The listing builds one solid part. Answer for the finished solid, in the listing's coordinates (mm). A direction names the side the tool comes from. Give positions to 0.01 mm unless a question says otherwise; leave off trailing zeros. Order: outer loops, then holes, each group sorted by start corner. A loop starts at its lowest first (then second) coordinate and runs counter-clockwise, first axis right, second up. Notation, with made-up numbers: (-29, -27) -> (15, -27) arc R27 ccw to (15, -4) -> close; hole circle Ø3 at (31, 7). An arc over 180 degrees is marked (long way). Write item = value, one per line. Start each with the question number.
```python
from build123d import *

# Parameters (mm, degrees)
PAD_DEPTH              = 30
SKETCH001_R            = 19
SKETCH001_R_2          = 5.5
POCKET_DEPTH           = 2
LINEARPATTERN_COUNT    = 2
LINEARPATTERN_PITCH    = 24
LINEARPATTERN001_COUNT = 2
LINEARPATTERN001_PITCH = 24
FILLET_R               = 5
CHAMFER_SIZE           = 0.5
CHAMFER001_SIZE        = 1


with BuildPart() as part:
    # Sketch → Pad (new body, symmetric)
    with BuildSketch(Plane.XZ):
        with BuildLine():
            ThreePointArc((-3.872983, 5), (0, 2), (3.872983, 5))
            Line((3.872983, 5), (7.872983, 5))
            Line((7.872983, 5), (9.994304, 2.87868))
            ThreePointArc((9.994304, 2.87868), (10.837449, 0.843146), (12.872983, 0))
            Line((30, 0), (12.872983, 0))
            Line((30, -3), (30, 0))
            Line((-30, -3), (30, -3))
            Line((-30, 0), (-30, -3))
            Line((-12.872983, 0), (-30, 0))
            ThreePointArc((-12.872983, 0), (-10.837449, 0.843146), (-9.994304, 2.87868))
            Line((-7.872983, 5), (-9.994304, 2.87868))
            Line((-3.872983, 5), (-7.872983, 5))
        make_face()
    extrude(amount=PAD_DEPTH, both=True)

    # Sketch001 → Pocket (cut, symmetric)
    with BuildSketch(Plane.XZ):
        with Locations((0, 18)):
            Circle(SKETCH001_R)
        with Locations((0, 6)):
            Circle(SKETCH001_R_2, mode=Mode.SUBTRACT)
    pocket = extrude(amount=POCKET_DEPTH, both=True, mode=Mode.SUBTRACT)

    # LinearPattern: Pocket ×2
    with Locations(*[(0, -i * LINEARPATTERN_PITCH, 0) for i in range(1, LINEARPATTERN_COUNT)]):
        add(pocket, mode=Mode.SUBTRACT)

    # LinearPattern001: Pocket ×2
    with Locations(*[(0, i * LINEARPATTERN001_PITCH, 0) for i in range(1, LINEARPATTERN001_COUNT)]):
        add(pocket, mode=Mode.SUBTRACT)

    # Fillet
    fillet_edges = [part.edges().sort_by_distance(p)[0] for p in [
        (30, -30, -1.5),
        (30, 30, -1.5),
        (-30, -30, -1.5),
        (-30, 30, -1.5),
    ]]
    fillet(fillet_edges, radius=FILLET_R)

    # Chamfer
    chamfer_edges = [part.edges().sort_by_distance(p)[0] for p in [
        (-5.872983, 30, 5),
        (-7.872983, 28, 5),
        (-6.640655, 26, 5),
        (-5.408327, 24, 5),
        (-6.640655, 22, 5),
        (-7.872983, 12, 5),
        (-6.640655, 2, 5),
        (-5.408327, 0, 5),
        (-6.640655, -2, 5),
        (-7.872983, -12, 5),
        (-6.640655, -22, 5),
        (-5.408327, -24, 5),
        (-6.640655, -26, 5),
        (-7.872983, -28, 5),
        (-5.872983, -30, 5),
        (-3.872983, 0, 5),
        (5.872983, 30, 5),
        (7.872983, 28, 5),
        (6.640655, 26, 5),
        (5.408327, 24, 5),
        (6.640655, 22, 5),
        (7.872983, 12, 5),
        (6.640655, 2, 5),
        (5.408327, 0, 5),
        (6.640655, -2, 5),
        (7.872983, -12, 5),
        (6.640655, -22, 5),
        (5.408327, -24, 5),
        (6.640655, -26, 5),
        (7.872983, -28, 5),
        (5.872983, -30, 5),
        (3.872983, 0, 5),
    ]]
    chamfer(chamfer_edges, length=CHAMFER_SIZE)

    # Chamfer001
    chamfer001_edges = [part.edges().sort_by_distance(p)[0] for p in [
        (18.936492, -30, 0),
        (-18.936492, -30, 0),
    ]]
    chamfer(chamfer001_edges, length=CHAMFER001_SIZE)


solid = part.part
```
Item 1: Consider L1, parallel to Y at x = -1, z = -0.75; L2, parallel to X at y = 23, z = 1.5; L3, parallel to Z at x = 22, y = -2. Determine where each line is inside the solid, lowest interval first. Write a range as from..to.
Item 2: A cutting plane is placed at B-B, the plane y = -15.5. Write down the section's boundary in (x, z), plus the area to 3 significant figures.
Item 3: Which of the six approach directions +Z, -Z, +X, -X, +Y, -Y give full straight-line access (tool end or side, diameter ignored) to faces 1 (the flat face through (21, 0, 0)), 2 (the flat face through (-30, 0, -2)), 3 (the flat face through (0, 2, 0)), 4 (the conical face through (10.37, 29.28, 0.95))?
Item 4: Flat-ended cylindrical pins translate along their axes: pin 1 (17.5 mm diameter, centred on x = 18, y = 8.5, fed in from +Z); pin 2 (8 mm diameter, centred on x = -21, y = -2.5, fed in from +Z). Find the tip coordinate at first contact, or state that the pin passes through.
Item 5: A cutting plane is placed at C-C, the plane x = 1. Write down the section's boundary in (y, z), plus the area to 3 significant figures.
Item 6: The mould has two halves that part along X. Classify faces 5 (the flat face through (-21, 0, 0)), 6 (the flat face through (9.098, -12.14, 3.775)), 7 (the flat face through (0, 26, 0)): +X half, -X half, draft (parallel to the pull), parting line (faces both ways), or undercut.
Item 7: A cutting plane is placed at A-A, the plane y = 23. Write down the section's boundary in (x, z).
Item 8: A cutting plane is placed at D-D, the plane z = 1.25. Count the separate pieces of the cut face and the enclosed holes in it, plus the area to 3 significant figures.
Check values:
q1.L1 = -30..-26, -22..-2, 2..22, 26..30
q1.L2 = -10.35..-9.42, -3.16..3.16, 9.42..10.35
q1.L3 = -3..0
q2.outline = (-30, -3) -> (30, -3) -> (30, -1) -> (29, 0) -> (12.87, 0) arc R2.88 cw to (9.99, 2.88) -> (8.23, 4.65) -> (7.37, 5) -> (4.37, 5) -> (3.72, 4.52) arc R4 cw to (-3.72, 4.52) -> (-4.37, 5) -> (-7.37, 5) -> (-8.23, 4.65) -> (-9.99, 2.88) arc R2.88 cw to (-12.87, 0) -> (-29, 0) -> (-30, -1) -> close
q2.area = 260 mm^2
q3.face_1 = +Z, +X, +Y, -Y
q3.face_2 = +Z, -Z, -X, +Y, -Y
q3.face_3 = none
q3.face_4 = +X, +Y
q4.pin_1 = 3.62
q4.pin_2 = 0
q5.outline = (-30, -3) -> (30, -3) -> (30, 2.13) -> (-30, 2.13) -> close; hole (-26, -0.97) -> (-22, -0.97) -> (-22, 0.59) -> (-26, 0.59) -> close; hole (-2, -0.97) -> (2, -0.97) -> (2, 0.59) -> (-2, 0.59) -> close; hole (22, -0.97) -> (26, -0.97) -> (26, 0.59) -> (22, 0.59) -> close
q5.area = 289 mm^2
q6.face_5 = draft
q6.face_6 = +X half
q6.face_7 = undercut
q7.outline = (-30, -3) -> (30, -3) -> (30, -1) -> (29, 0) -> (12.87, 0) arc R2.88 cw to (10.15, 1.94) arc R19 cw to (-10.15, 1.94) arc R2.88 cw to (-12.87, 0) -> (-29, 0) -> (-30, -1) -> close; (-5.3, 4.51) arc R5.5 ccw to (5.3, 4.51) -> (4.91, 5) -> (4.37, 5) -> (3.72, 4.52) arc R4 cw to (-3.72, 4.52) -> (-4.37, 5) -> (-4.91, 5) -> close
q8.separate_pieces = 1
q8.enclosed_holes = 6
q8.area = 1,110 mm^2
